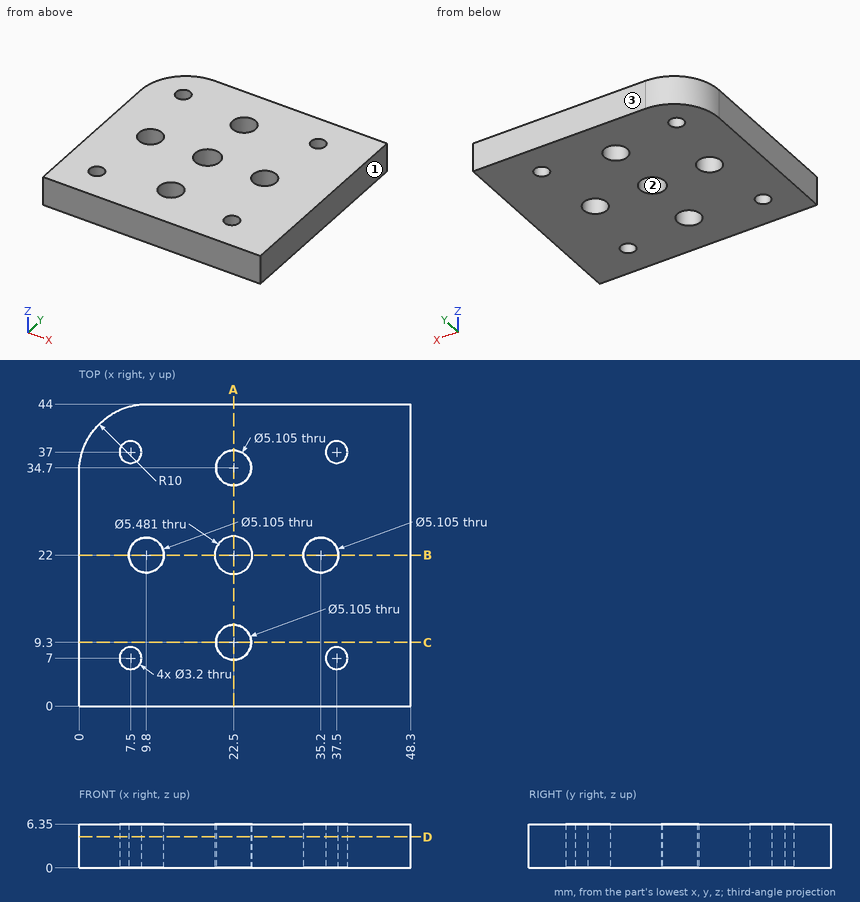
Source: three-view drawing plus pictorial views. Frame: mm from the lowest corner of the part. Round coordinates to 2 decimals unless told otherwise and drop trailing zeros. Loops run counter-clockwise (first coordinate to the right, second up) from the corner with the lowest first, then second, coordinate; pieces in that order, holes last. Notation, with made-up numbers: (14, 11.5) -> (25, 11.5) arc R22 cw to (25, 41.5) -> close; hole circle Ø5 at (-21, 11). An arc over 180 degrees is marked (long way). Use one line per item in the form item = value.
Item 1: Cut plane A-A on x = 22.5. Output: boundary loops of the cut face in (y, z), then the cut area to 3 significant figures.
Evaluation:
outline = (0, 0) -> (6.75, 0) -> (6.75, 6.35) -> (0, 6.35) -> close; (11.85, 0) -> (19.26, 0) -> (19.26, 6.35) -> (11.85, 6.35) -> close; (24.74, 0) -> (32.15, 0) -> (32.15, 6.35) -> (24.74, 6.35) -> close; (37.25, 0) -> (44, 0) -> (44, 6.35) -> (37.25, 6.35) -> close
area = 180 mm2
Item 2: Cut plane B-B on y = 22. Output: boundary loops of the cut face in (x, z).
Evaluation:
outline = (0, 0) -> (7.25, 0) -> (7.25, 6.35) -> (0, 6.35) -> close; (12.35, 0) -> (19.76, 0) -> (19.76, 6.35) -> (12.35, 6.35) -> close; (25.24, 0) -> (32.65, 0) -> (32.65, 6.35) -> (25.24, 6.35) -> close; (37.75, 0) -> (48.3, 0) -> (48.3, 6.35) -> (37.75, 6.35) -> close
Item 3: Draft query along Y for the marked faces 1, 2 and 3. Return one class per face: released by +Y, released by -Y, zero draft, split by the parting line, or undercut.
Evaluation:
face_1 = zero draft
face_2 = undercut
face_3 = released by +Y
Item 4: Cut plane C-C on y = 9.3. Output: boundary loops of the cut face in (x, z), then the cut area to 3 significant figures.
Evaluation:
outline = (0, 0) -> (19.95, 0) -> (19.95, 6.35) -> (0, 6.35) -> close; (25.05, 0) -> (48.3, 0) -> (48.3, 6.35) -> (25.05, 6.35) -> close
area = 274 mm2
Item 5: Cut plane D-D on z = 4.5. Give the number of separate pieces and of enclosed holes in the cut face, then the cut area to 3 significant figures.
Evaluation:
separate_pieces = 1
enclosed_holes = 9
area = 1,970 mm2
Item 6: Material intervals for probe 1 along Y at (x, z) = (22.5, 3.75); probe 2 along Y at (x, z) = (37.5, 4.25) (1 decimal); probe 3 along Y at (x, z) = (7, 2.75), sorted ascending.
Evaluation:
probe_1 = 0 to 6.75, 11.85 to 19.26, 24.74 to 32.15, 37.25 to 44
probe_2 = 0 to 5.4, 8.6 to 20.9, 23.1 to 35.4, 38.6 to 44
probe_3 = 0 to 5.48, 8.52 to 35.48, 38.52 to 43.54
